Check sheet for the modelled part. Datum: model origin and axes. Units: mm. Face numbers are marked on the shaded views. A direction names the side the tool comes from. Round coordinates to 2 decimals unless told otherwise and drop trailing zeros. Order: outer loops, then holes, each group sorted by start corner. A loop starts at its lowest first (then second) coordinate and runs counter-clockwise, first axis right, second up.
(1) Sectioned sample at B-B, the plane y = 23. Enter the section's corners in (x, z), and give its area (3 significant figures).
(2) Sectioned sample at C-C, the plane x = 10. Enter the section's corners in (y, z) (3 decimals), and give its area (3 significant figures).
(3) Depth check by flat-ended pin: pin 1 (12 mm diameter, centred on x = 39.5, y = 22.5, fed in from +Z); pin 2 (12 mm diameter, centred on x = 61.5, y = 41.5, fed in from +Z); pin 3 (8.5 mm diameter, centred on x = 28, y = 48, fed in from +Z). Enter the tip coordinate at first touch or a pass-through.
(4) Tool access check on the marked faces 4 and 5. Record the directions out of +Z, -Z, +X, -X, +Y, -Y that give a thin tool (end or side, any length) a straight path to the whole face; none if there is none.
(5) Sectioned sample at A-A, the plane y = 6.05. Count the separate pieces of the cut face and the enclosed holes in it, and give its area (3 significant figures).
(6) Mould release check, pull along X, two halves, no side actions. Record for the marked faces 1, 2 and 3: released by +X, released by -X, zero draft, split by the parting line, or undercut.
(7) Thickness scan on probe 1 along X at (y, z) = (3, 3.75); probe 2 along Y at (x, z) = (79, 1.4) (3 decimals); probe 3 along X at (y, z) = (33.5, 3.5). Record the ranges inside material, lowest first.
(8) Sectioned sample at D-D, the plane z = 13.75. Enter the section's corners in (x, y), and give its area (3 significant figures).
Autodesk Fusion 360 part; units mm, degrees
sketch "Sketch1" plane through (0, 0, 0) normal (0, 0, 1) x (1, 0, 0)
  line L0 (0, 0) -> (5, 0)
  line L1 (5, 0) -> (5, 37.75)
  line L2 (0, 52.75) -> (0, 0)
  line L3 (51, 37.75) -> (51, 0)
  line L4 (51, 0) -> (56, 0)
  line L5 (56, 0) -> (56, 37.75)
  line L6 (102, 37.75) -> (102, 0)
  line L7 (102, 0) -> (107, 0)
  line L8 (107, 0) -> (107, 37.75)
  line L9 (153, 37.75) -> (153, 0)
  line L10 (153, 0) -> (158, 0)
  line L11 (158, 0) -> (158, 52.75)
  line L12 (0, 52.75) -> (158, 52.75)
  line L13 (51, 37.75) -> (5, 37.75)
  line L14 (153, 37.75) -> (107, 37.75)
  line L15 (102, 37.75) -> (56, 37.75)
  line L16 (0, 45.25) -> (158, 45.25) construction
  circle A0 centre (10, 45.25) radius 1.625
  circle A1 centre (79, 45.25) radius 1.625
  circle A2 centre (148, 45.25) radius 1.625
  dimension "d2" = 52.75
  dimension "d10" = 7.5
  dimension "d11" = 3.25
  dimension "d12" = 10
  dimension "d13" = 10
  dimension "d25" = 15
extrude "Extrude1" add sketch "Sketch1" along normal blind 3.5 makes body 1
sketch "Sketch2" plane through (0, 0, 0) normal (-1, 0, 0) x (0, -1, 0)
  line L0 (-52.75, 0) -> (0, 0)
  line L1 (0, 0) -> (0, 3.5)
  line L2 (0, 3.5) -> (-52.75, 3.5)
  line L3 (-52.75, 3.5) -> (-52.75, 0)
  line L4 (0, 3.5) -> (0, 15.5)
  line L5 (0, 15.5) -> (-25, 15.5)
  line L6 (0, 9.5) -> (-18.95, 9.5) construction
  circle A0 centre (-6.05, 9.5) radius 1.75
  circle A1 centre (-18.95, 9.5) radius 1.75
  line L7 (-25, 15.5) -> (-52.75, 3.5)
  dimension "d16" = 25
  dimension "d19" = 9.5
  dimension "d20" = 3.5
  dimension "d23" = 6.05
  dimension "d24" = 12.9
  dimension "d26" = 15.5
extrude "Extrude2" add sketch "Sketch2" against normal blind 5 separate body contours L2 L4 L5 L7 makes body 2
pattern_linear "R-Pattern1" count 4 spacing 51 along (1, 0, 0) of bodies 2 makes body 3 at (51, 32.7908, 9.3281) makes body 4 at (102, 32.7908, 9.3281) makes body 5 at (153, 32.7908, 9.3281)
combine "Combine1" operation add target body 1 tool bodies 2 3 4 5
fillet "Fillet2" radius 7.5 6 edges at (5, 37.75, 1.75) (51, 37.75, 1.75) (56, 37.75, 1.75) (102, 37.75, 1.75) (107, 37.75, 1.75) (153, 37.75, 1.75) on bodies 1
fillet "Fillet3" radius 2.5 6 edges at (102, 41.5, 3.5) (51, 41.5, 3.5) (153, 41.5, 3.5) (5, 41.5, 3.5) (56, 41.5, 3.5) (107, 41.5, 3.5) on bodies 1
sketch "Sketch3" plane through (158, 0, 0) normal (1, 0, 0) x (0, 1, 0)
  circle A0 centre (6.05, 9.5) radius 1.75
  circle A1 centre (18.95, 9.5) radius 1.75
  line L0 (0, 0) -> (52.75, 0)
  line L1 (52.75, 0) -> (52.75, 3.5)
  line L2 (52.75, 3.5) -> (25, 15.5)
  line L3 (25, 15.5) -> (0, 15.5)
  line L4 (0, 15.5) -> (0, 0)
  line L5 (6.05, 9.5) -> (18.95, 9.5) construction
  line L6 (12.5, 9.5) -> (12.5, 3.5) construction
  line L7 (10, 2.5) -> (15, 2.5)
  arc A2 (15, 2.5) -> (15, 4.5) centre (15, 3.5) ccw
  line L8 (15, 4.5) -> (10, 4.5)
  arc A3 (10, 4.5) -> (10, 2.5) centre (10, 3.5) ccw
  line L9 (10, 3.5) -> (15, 3.5) construction
  point P0 (12.5, 3.5)
  dimension "d39" = 3.5
  dimension "d40" = 2.5
  dimension "d41" = 1
extrude "Extrude3" cut sketch "Sketch3" against normal blind 160 contours L7 A2 L8 A3 bodies 1
equation "d2 = 36.25 mm + 15 mm + 1.5 mm"
equation "d23 = 4.55 mm + 1.5 mm"
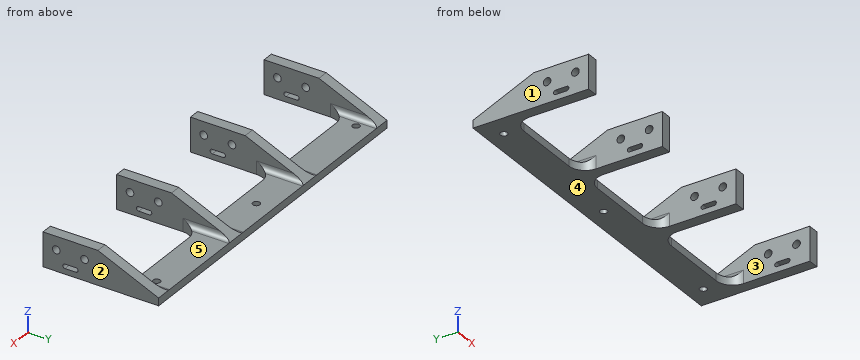
Derived:
1. outline: (0, 0) - (5, 0) - (5, 15.5) - (0, 15.5) - close; (51, 0) - (56, 0) - (56, 15.5) - (51, 15.5) - close; (102, 0) - (107, 0) - (107, 15.5) - (102, 15.5) - close; (153, 0) - (158, 0) - (158, 15.5) - (153, 15.5) - close
1. area: 310 mm2
2. outline: (37.321, 0) - (43.625, 0) - (43.625, 3.5) - (37.321, 3.5) - close; (46.875, 0) - (52.75, 0) - (52.75, 3.5) - (46.875, 3.5) - close
2. area: 42.6 mm2
3. pin 1: passes through
3. pin 2: stops at z = 9.4
3. pin 3: stops at z = 3.5
4. face 4: -Z, +X, -X, +Y, -Y
4. face 5: +Z, +Y, -Y
5. separate pieces: 8
5. enclosed holes: 0
5. area: 240 mm2
6. face 1: released by -X
6. face 2: released by +X
6. face 3: undercut
7. probe 1: x = 0 to 5, 51 to 56, 102 to 107, 153 to 158
7. probe 2: y = 37.75 to 43.625, 46.875 to 52.75
7. probe 3: x = 0 to 5.74, 50.26 to 56.74, 101.26 to 107.74, 152.26 to 158
8. outline: (0, 0) - (5, 0) - (5, 29.05) - (0, 29.05) - close; (51, 0) - (56, 0) - (56, 29.05) - (51, 29.05) - close; (102, 0) - (107, 0) - (107, 29.05) - (102, 29.05) - close; (153, 0) - (158, 0) - (158, 29.05) - (153, 29.05) - close
8. area: 581 mm2
